For this review, use the dimensioned drawing (mm, ordinates from the lowest corner) and the shaded views. A direction names the side the tool comes from. Round coordinates to 2 decimals unless told otherwise and drop trailing zeros. Loops run counter-clockwise (first coordinate to the right, second up) from the corner with the lowest first, then second, coordinate; pieces in that order, holes last. Notation, with made-up numbers: (38.25, 43.25) -> (78.25, 43.25) arc R35 cw to (78.25, 79.25) -> close; hole circle Ø2 at (33.25, 40). An arc over 180 degrees is marked (long way). Answer as CSV lines item,"result". Start each with the question number.
(1) Take a section at B-B, the plane z = 5. Write out the cut boundary in (x, y), and give its area (3 significant figures).
(2) Take a section at A-A, the plane y = 10. Write out the cut boundary in (x, z), and give its area (3 significant figures).
(3) Take a section at D-D, the plane x = 2. Write out the cut boundary in (y, z).
(4) To check wall thickness, follow line 1 (X direction, y = 0.8, z = 5); line 2 (X direction, y = 9.5, z = 1.25). State the ranges of each line that lie inside material, in increasing order. Write a range as from..to.
(5) For P1, Ø3.5, axis at x = 10, z = 5, coming from the +Y side; P2, Ø2.5, axis at y = 10, z = 5, coming from the -X side; P3, Ø2, axis at y = 10.5, z = 6, coming from the +X side; P4, Ø7.5, axis at x = 11, z = 11.5, coming from the +Y side, all flat-tipped, find the tip position at first contact; note any pin that passes through.
(6) Machinability: for the marked faces 5 and 6, which of the approach directions +Z, -Z, +X, -X, +Y, -Y give a long, thin tool a straight path to every point of the face, cutting with its end or side? Answer none if there is none.
(7) Draft analysis for pull direction Z (two halves, no side actions). For the marked faces 1, 2, 3 and 4, state which applies: +Z half, -Z half, draft (parallel to the pull), parting line (faces both ways), or undercut.
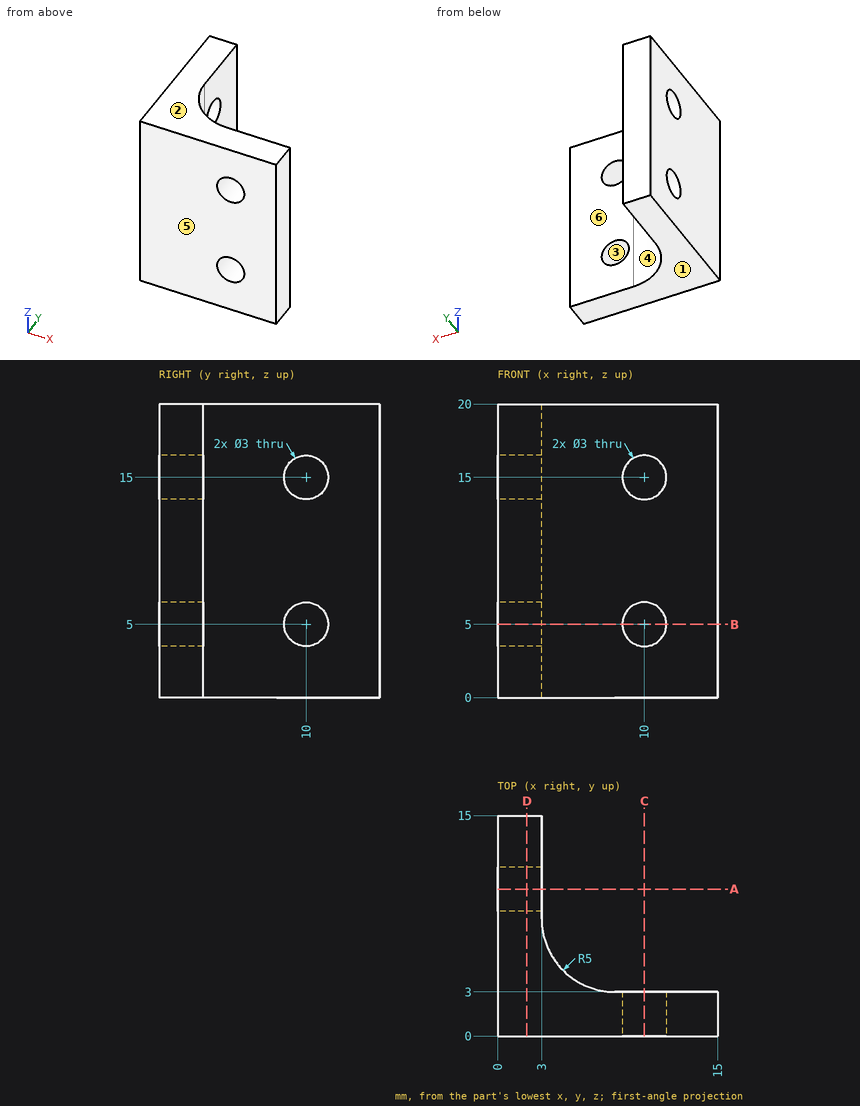
The answers:
1,outline,"(0, 0) -> (8.5, 0) -> (8.5, 3) -> (8, 3) arc R5 cw to (3, 8) -> (3, 8.5) -> (0, 8.5) -> close; (0, 11.5) -> (3, 11.5) -> (3, 15) -> (0, 15) -> close; (11.5, 0) -> (15, 0) -> (15, 3) -> (11.5, 3) -> close"
1,area,"68.4 mm²"
2,outline,"(0, 0) -> (3, 0) -> (3, 3.5) -> (0, 3.5) -> close; (0, 6.5) -> (3, 6.5) -> (3, 13.5) -> (0, 13.5) -> close; (0, 16.5) -> (3, 16.5) -> (3, 20) -> (0, 20) -> close"
2,area,"42.0 mm²"
3,outline,"(0, 0) -> (15, 0) -> (15, 20) -> (0, 20) -> close; hole circle Ø3 at (10, 5); hole circle Ø3 at (10, 15)"
4,line 1,"0..8.5, 11.5..15"
4,line 2,"0..3"
5,P1,"y = 3"
5,P2,"through"
5,P3,"x = 3"
5,P4,"y = 3.06"
6,face 5,"+Z, -Z, +X, -X, -Y"
6,face 6,"+Z, -Z, +X, +Y"
7,face 1,"-Z half"
7,face 2,"+Z half"
7,face 3,"undercut"
7,face 4,"draft"
